```python
from build123d import *

# Parameters (mm, degrees)
PAD_DEPTH       = 15
SKETCH022_W     = 3
SKETCH022_H     = 2
PAD003_DEPTH    = 4.5
SKETCH024_W     = 14
SKETCH024_H     = 14
POCKET001_DEPTH = 5
SKETCH025_W     = 6.3
SKETCH025_H     = 10
POCKET002_DEPTH = 5.001
SKETCH028_R     = 1.55
POCKET005_DEPTH = 20.701
POCKET006_DEPTH = 4
CHAMFER001_SIZE = 2
FILLET001_R     = 2
FILLET006_R     = 1
FILLET008_R     = 1
FILLET009_R     = 3
FILLET010_R     = 2
PAD005_DEPTH    = 10
FILLET011_R     = 5


with BuildPart() as part:
    # Sketch → Pad (new body, symmetric)
    with BuildSketch(Plane.XZ):
        Polygon((0, 0), (10, 0), (10, 20.7), (3.4, 20.7), (3.4, 15.5), (2, 15.5), (2, 14), (1, 15), (0, 15), align=None)
    extrude(amount=PAD_DEPTH, both=True)

    # Sketch022 → Pad003 (new body)
    with BuildSketch(Plane(origin=(0, 0, 20.7), x_dir=(-1, 0, 0), z_dir=(0, 0, 1))):
        with Locations((-8.5, 14)):
            Rectangle(SKETCH022_W, SKETCH022_H)
        with Locations((-8.5, -14)):
            Rectangle(SKETCH022_W, SKETCH022_H)
    extrude(amount=PAD003_DEPTH)

    # Sketch024 → Pocket001 (cut)
    with BuildSketch(Plane(origin=(10, 0, 0), x_dir=(0, 0, 1), z_dir=(1, 0, 0))):
        with Locations((13.7, 0)):
            Rectangle(SKETCH024_W, SKETCH024_H)
    extrude(amount=-POCKET001_DEPTH, mode=Mode.SUBTRACT)

    # Sketch025 → Pocket002 (cut, through all)
    with BuildSketch(Plane(origin=(5, 0, 0), x_dir=(0, 0, 1), z_dir=(1, 0, 0))):
        with Locations((17.55, 0)):
            Rectangle(SKETCH025_W, SKETCH025_H)
    extrude(amount=-POCKET002_DEPTH, mode=Mode.SUBTRACT)

    # Sketch028 → Pocket005 (cut, through all)
    with BuildSketch(Plane(origin=(0, 0, 20.7), x_dir=(-1, 0, 0), z_dir=(0, 0, 1))):
        with Locations((-6.5, 10)):
            Circle(SKETCH028_R)
        with Locations((-6.5, -10)):
            Circle(SKETCH028_R)
    extrude(amount=-POCKET005_DEPTH, mode=Mode.SUBTRACT)

    # Sketch029 → Pocket006 (cut)
    with BuildSketch(Plane(origin=(0, 0, 0), x_dir=(1, 0, 0), z_dir=(0, 0, -1))):
        Polygon((9.3, 11.616581), (9.3, 8.383419), (6.5, 6.766838), (3.7, 8.383419), (3.7, 11.616581), (6.5, 13.233162), align=None)
        Polygon((6.5, -6.766838), (9.3, -8.383419), (9.3, -11.616581), (6.5, -13.233162), (3.7, -11.616581), (3.7, -8.383419), align=None)
    extrude(amount=-POCKET006_DEPTH, mode=Mode.SUBTRACT)

    # Chamfer001
    chamfer001_edges = [part.edges().sort_by_distance(p)[0] for p in [
        (5, 0, 14.4),
    ]]
    chamfer(chamfer001_edges, length=CHAMFER001_SIZE)

    # Fillet001
    fillet001_edges = [part.edges().sort_by_distance(p)[0] for p in [
        (3, 0, 14.4),
    ]]
    fillet(fillet001_edges, radius=FILLET001_R)

    # Fillet006
    fillet006_edges = [part.edges().sort_by_distance(p)[0] for p in [
        (0, 0, 14.4),
    ]]
    fillet(fillet006_edges, radius=FILLET006_R)

    # Fillet008
    fillet008_edges = [part.edges().sort_by_distance(p)[0] for p in [
        (2, -15, 14.75),
        (1.5, -15, 14.5),
        (1.5, 15, 14.5),
        (2, 15, 14.75),
    ]]
    fillet(fillet008_edges, radius=FILLET008_R)

    # Fillet009
    fillet009_edges = [part.edges().sort_by_distance(p)[0] for p in [
        (3.4, -15, 18.1),
        (3.4, 15, 18.1),
    ]]
    fillet(fillet009_edges, radius=FILLET009_R)

    # Fillet010
    fillet010_edges = [part.edges().sort_by_distance(p)[0] for p in [
        (10, 0, 6.7),
    ]]
    fillet(fillet010_edges, radius=FILLET010_R)

    # Sketch030 → Pad005 (new body)
    with BuildSketch(Plane(origin=(10, 0, 0), x_dir=(0, 0, 1), z_dir=(1, 0, 0))):
        Polygon((3, 15), (10, 15), (3, 17), align=None)
        Polygon((3, -17), (10, -15), (3, -15), align=None)
    extrude(amount=-PAD005_DEPTH)

    # Fillet011
    fillet011_edges = [part.edges().sort_by_distance(p)[0] for p in [
        (5, -15, 10),
        (5, 15, 10),
    ]]
    fillet(fillet011_edges, radius=FILLET011_R)


solid = part.part
```
Geometry check sheet. Reference: the model listing, model coordinates, mm. A direction names the side the tool comes from. Coordinates: 2 decimals unless noted, no trailing zeros. Write each loop counter-clockwise with the first axis right and the second up, starting at its lowest first coordinate (ties: lowest second). Pieces come first, ordered by that corner, then holes. Notation, with made-up numbers: M 70.5,-32.5 L 123.5,-32.5 A21 cw 123.5,-6.5 Z; hole C -14.5,5 d3. An arc over 180 degrees is marked long. Answer as a JSON object with one key per item and string values.
1. Section check A-A, the plane z = 18.5. Enter the section's corners in (x, y), plus the area to 3 significant figures.
Answers below:
{"outline": "M 3.4,-12 A3 ccw 6.4,-15 L 10,-15 L 10,-7 L 5,-7 L 5,-5 L 3.4,-5 Z; M 3.4,5 L 5,5 L 5,7 L 10,7 L 10,15 L 6.4,15 A3 ccw 3.4,12 Z; hole C 6.5,-10 d3.1; hole C 6.5,10 d3.1", "area": "93.0 mm²"}
2. Section check D-D, the plane z = 5.5. Enter the section's corners in (x, y), plus the area to 3 significant figures.
Answers below:
{"outline": "M 0,-16.29 L 10,-16.29 L 10,-7 L 9.83,-7 L 9.83,7 L 10,7 L 10,16.29 L 0,16.29 Z; hole C 6.5,-10 d3.1; hole C 6.5,10 d3.1", "area": "308 mm²"}
3. Section check B-B, the plane y = 10. Enter the section's corners in (x, z).
Answers below:
{"outline": "M 0,0 L 3.7,0 L 3.7,4 L 4.95,4 L 4.95,20.7 L 3.4,20.7 L 3.4,15.5 L 2,15.5 L 2,14 L 1,15 L 0,15 Z; M 8.05,4 L 9.3,4 L 9.3,0 L 10,0 L 10,20.7 L 8.05,20.7 Z"}
4. Go/stop test with flat-tipped pins: pin 1 Ø1.5 at (y, z) = (4, 22.5) entering from +X; pin 2 Ø4 at (x, y) = (6.5, -10) entering from -Z; pin 3 Ø2.5 at (x, z) = (7.5, 10) entering from +Y; pin 4 Ø1.3 at (x, y) = (5, 12) entering from +Z. Record where each tip stops, or that it passes through.
Answers below:
{"pin 1": "passes through", "pin 2": "stops at z = 4", "pin 3": "stops at y = 15.36", "pin 4": "stops at z = 20.7"}
5. Tool access check on faces 1 (the cylindrical face through (4.3, 14.14, 18.06)), 2 (the flat face through (7, 0, 6.7)), 3 (the flat face through (5, 11, 4)), 4 (the flat face through (5, -16, 3)). Record the directions out of +Z, -Z, +X, -X, +Y, -Y that give a thin tool (end or side, any length) a straight path to the whole face; none if there is none.
Answers below:
{"face 1": "+Z, -X, +Y", "face 2": "+Z, +X", "face 3": "-Z", "face 4": "-Z, +X, -X, -Y"}
6. Draft check along X on faces 5 (the cylindrical face through (1.43, 14.813, 13.98)), 6 (the flat face through (9, -14, 25.2)), 7 (the cylindrical face through (2.4, 14.8, 14.4)), 8 (the flat face through (5, 0, 10)). Enter one of: released by +X, released by -X, zero draft, split by the parting line, or undercut.
Answers below:
{"face 5": "undercut", "face 6": "zero draft", "face 7": "undercut", "face 8": "released by +X"}
7. Scan lines: L1, parallel to Y at x = 6.5, z = 15; L2, parallel to X at y = 10, z = 17; L3, parallel to Y at x = 9, z = 12.75. Record each from-to range of solid material in increasing order.
Answers below:
{"L1": "y = -15 to -11.55, -8.45 to -7, 7 to 8.45, 11.55 to 15", "L2": "x = 3.4 to 4.95, 8.05 to 10", "L3": "y = -15 to -7, 7 to 15"}
8. Section check C-C, the plane y = -0.5. Enter the section's corners in (x, z), plus the area to 3 significant figures.
Answers below:
{"outline": "M 0,0 L 10,0 L 10,4.7 A2 ccw 8,6.7 L 5,6.7 L 5,12.4 L 3.59,13.81 A2 ccw 2.17,14.4 L 2,14.4 L 2,14 L 1.6,14.4 L 1,14.4 A1 ccw 0,13.4 Z", "area": "102 mm²"}
